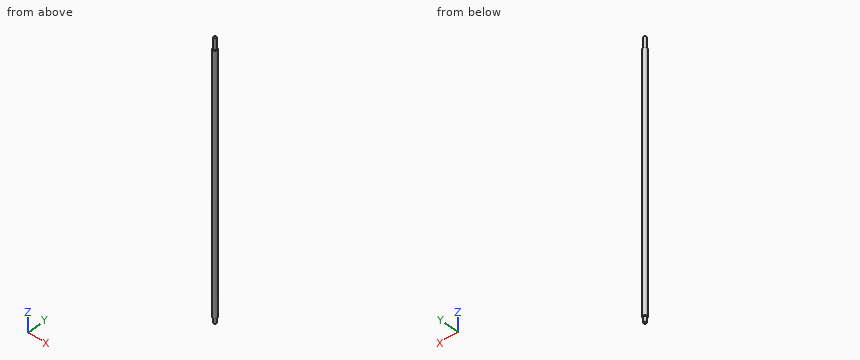
```python
from build123d import *

# Parameters (mm, degrees)
SKETCH1_R           = 4.7625
BOSS_EXTRUDE1_DEPTH = 609.6
CUT_EXTRUDE1_START  = -25.4
SKETCH2_R           = 4.7625
SKETCH2_R_2         = 3.0607
CUT_EXTRUDE1_DEPTH  = 25.4
SKETCH3_R           = 4.7625
SKETCH3_R_2         = 3.0607
CUT_EXTRUDE3_DEPTH  = 12.7


with BuildPart() as part:
    # Sketch1 → Boss-Extrude1 (new body)
    with BuildSketch(Plane.XY):
        with Locations(Location((0, 0, 0), (0, 0, 180))):
            Circle(SKETCH1_R)
    extrude(amount=BOSS_EXTRUDE1_DEPTH)

    # Sketch2 → Cut-Extrude1 (cut)
    with BuildSketch(Plane.XY.offset(609.6).offset(CUT_EXTRUDE1_START)):
        with Locations(Location((0, 0, 0), (0, 0, 180))):
            Circle(SKETCH2_R)
        Circle(SKETCH2_R_2, mode=Mode.SUBTRACT)
    extrude(amount=CUT_EXTRUDE1_DEPTH, mode=Mode.SUBTRACT)

    # Sketch3 → Cut-Extrude3 (cut)
    with BuildSketch(Plane(origin=(0, 0, 0), x_dir=(-1, 0, 0), z_dir=(0, 0, -1))):
        Circle(SKETCH3_R)
        with Locations(Location((0, 0, 0), (0, 0, 180))):
            Circle(SKETCH3_R_2, mode=Mode.SUBTRACT)
    extrude(amount=-CUT_EXTRUDE3_DEPTH, mode=Mode.SUBTRACT)


solid = part.part
```
Geometry check sheet. Reference: the model listing, model coordinates, mm. Round coordinates to 2 decimals unless told otherwise and drop trailing zeros. Loops run counter-clockwise (first coordinate to the right, second up) from the corner with the lowest first, then second, coordinate; pieces in that order, holes last. Notation, with made-up numbers: (66, 59.25) - (122, 59.25) arc R13 cw to (122, 68.25) - close; hole circle Ø6 at (71, 64.25). An arc over 180 degrees is marked (long way). Use a Markdown table: item, result.
Q1. Go/stop test with flat-tipped pins: P1, Ø1.5, axis at y = -1.5, z = 151, coming from the -X side; P2, Ø3, axis at x = 3, y = 4, coming from the -Z side. Record where each tip stops, or that it passes through.
Solutions:
| item | result |
|---|---|
| P1 | stops at x = -4.7 |
| P2 | stops at z = 12.7 |
Q2. Material ranges on line 1 (Z direction, x = 0.75, y = -3); line 2 (X direction, y = -0.75, z = 372), recorded low to high.
Solutions:
| item | result |
|---|---|
| line 1 | z = 12.7 to 584.2 |
| line 2 | x = -4.7 to 4.7 |
Q3. Cross-section at A-A on x = 0. Record the cut outline in (y, z).
Solutions:
| item | result |
|---|---|
| outline | (-4.76, 12.7) - (-3.06, 12.7) - (-3.06, 0) - (3.06, 0) - (3.06, 12.7) - (4.76, 12.7) - (4.76, 584.2) - (3.06, 584.2) - (3.06, 609.6) - (-3.06, 609.6) - (-3.06, 584.2) - (-4.76, 584.2) - close |
Q4. Cross-section at C-C on z = 117.5. Record the cut outline in (x, y) (1 decimal).
Solutions:
| item | result |
|---|---|
| outline | circle Ø9.5 at (0, 0) |
